Geometry: final body of the model. Coordinates: model frame, mm. A direction names the side the tool comes from. Give positions to 0.01 mm unless a question says otherwise; leave off trailing zeros. Loops run counter-clockwise (first coordinate to the right, second up) from the corner with the lowest first, then second, coordinate; pieces in that order, holes last.
1. First-contact query: P1, Ø3, axis at y = 44, z = 3, coming from the -X side; P2, Ø4, axis at x = 67, y = 6.5, coming from the -Z side; P3, Ø5.5, axis at x = 65.31, y = 5.53, coming from the -Z side. Flat tips, straight axial feed; report the tip coordinate or a pass-through.
2. Section D-D, the plane x = 58. Output: boundary loops of the cut face in (y, z), then the cut area to 3 significant figures.
3. Section C-C, the plane z = 2. Output: boundary loops of the cut face in (x, y), then the cut area to 3 significant figures.
4. Section A-A, the plane x = 38. Output: boundary loops of the cut face in (y, z), then the cut area to 3 significant figures.
5. Section B-B, the plane y = 6.5. Output: boundary loops of the cut face in (x, z).
6. Draft query along X for faces 1 (the face through (35.42, 70, 3)), 2 (the face through (69, 38, 0)), 3 (the face through (67.005, 6.066, 5.584)). Return one class per face: +X half, -X half, draft (parallel to the pull), parting line (faces both ways), or undercut.
7. Material intervals for line 1 along Y through (x, z) = (62.5, 1.75); line 2 along Y through (x, z) = (64, 1.25); line 3 along Y through (x, z) = (39.5, 4.75), sorted ascending.
8. Access query for faces 4 (the face through (35.42, 1, 3)), 5 (the face through (64, 4, 4.039)). Directions: +Z, -Z, +X, -X, +Y, -Y. A direction counts if a zero-diameter tool reaches every point of the face in a straight line with its end or side. Return the directions, or none.
from build123d import *

# Parameters (mm, degrees)
F0_R     = 3.81
F1_DEPTH = 7.0866
F2_R     = 1.778
F2_R_2   = 3.81
F3_DEPTH = 3.048
F4_DEPTH = 25.4


with BuildPart() as f1:
    # F0 (on Top) → F1 (new body)
    with BuildSketch(Plane.XY):
        with BuildLine():
            Line((35.4203, 1.9812), (35.4203, 0))
            Line((35.4203, 0), (70.8406, 0))
            Line((70.8406, 0), (70.8406, 70.8406))
            Line((70.8406, 70.8406), (35.4203, 70.8406))
            Line((35.4203, 70.8406), (35.4203, 68.8594))
            ThreePointArc((35.4203, 68.8594), (68.8594, 35.4203), (35.4203, 1.9812))
        make_face()
        with Locations((65.308762, 5.531838)):
            Circle(F0_R, mode=Mode.SUBTRACT)
        with Locations((65.308762, 65.308762)):
            Circle(F0_R, mode=Mode.SUBTRACT)
    extrude(amount=F1_DEPTH)

    # F2 (on face) → F3 (join)
    with BuildSketch(Plane.XY.offset(7.0866)):
        with Locations((65.308762, 5.531838)):
            Circle(F2_R)
        with Locations((65.308762, 65.308762)):
            Circle(F2_R)
        with Locations((65.308762, 65.308762)):
            Circle(F2_R_2)
        with Locations((65.308762, 65.308762)):
            Circle(F2_R, mode=Mode.SUBTRACT)
        with Locations((65.308762, 5.531838)):
            Circle(F2_R_2)
        with Locations((65.308762, 5.531838)):
            Circle(F2_R, mode=Mode.SUBTRACT)
    extrude(amount=-F3_DEPTH)

    # F2 (on face) → F4 (cut)
    with BuildSketch(Plane.XY.offset(7.0866)):
        with Locations((65.308762, 5.531838)):
            Circle(F2_R)
        with Locations((65.308762, 65.308762)):
            Circle(F2_R)
    extrude(amount=-F4_DEPTH, mode=Mode.SUBTRACT)


solid = f1.part
Answers below:
1. P1: stops at x = 67.3
1. P2: stops at z = 0
1. P3: stops at z = 4.04
2. outline: (0, 0) - (10.76, 0) - (10.76, 7.09) - (0, 7.09) - close; (60.08, 0) - (70.84, 0) - (70.84, 7.09) - (60.08, 7.09) - close
2. area: 152 mm2
3. outline: (35.42, 0) - (70.84, 0) - (70.84, 70.84) - (35.42, 70.84) - (35.42, 68.86) arc R33.44 cw to (35.42, 1.98) - close; hole circle Ø7.62 at (65.31, 5.53); hole circle Ø7.62 at (65.31, 65.31)
3. area: 662 mm2
4. outline: (0, 0) - (2.08, 0) - (2.08, 7.09) - (0, 7.09) - close; (68.76, 0) - (70.84, 0) - (70.84, 7.09) - (68.76, 7.09) - close
4. area: 29.5 mm2
5. outline: (52.21, 0) - (61.62, 0) - (61.62, 4.04) - (63.82, 4.04) - (63.82, 7.09) - (52.21, 7.09) - close; (66.8, 4.04) - (68.99, 4.04) - (68.99, 0) - (70.84, 0) - (70.84, 7.09) - (66.8, 7.09) - close
6. face 1: -X half
6. face 2: draft
6. face 3: undercut
7. line 1: y = 0 to 2.96, 8.11 to 15.8, 55.04 to 62.73, 67.88 to 70.84
7. line 2: y = 0 to 1.95, 9.11 to 18.06, 52.78 to 61.73, 68.89 to 70.84
7. line 3: y = 0 to 2.23, 68.61 to 70.84
8. face 4: +Z, -Z, -X, +Y, -Y
8. face 5: -Z
